For this review, take the finished solid that the model builds, in its own axes (mm). A direction names the side the tool comes from. Round coordinates to 2 decimals unless told otherwise and drop trailing zeros. Loops run counter-clockwise (first coordinate to the right, second up) from the corner with the lowest first, then second, coordinate; pieces in that order, holes last. Notation, with made-up numbers: M 41,51 L 78,51 A18 ccw 78,84 Z; hole C 13.5,-5.5 d2. An arc over 180 degrees is marked long. One line per question, with ' | ' between items. Start each with the question number.
1) We need section B-B (x = -10). Give the boundary of the cut face in (y, z).
2) We need section D-D (y = -2.5). Give the boundary of the cut face in (x, z), and give its area (3 significant figures).
3) We need section A-A (y = 3). Give the boundary of the cut face in (x, z), and give its area (3 significant figures).
4) We need section C-C (z = 5). Give the boundary of the cut face in (x, y), and give its area (3 significant figures).
5) Mouldability with a two-part tool opening along Y and no side actions: class faces 3 (the face through (5, 0, 8)), 4 (the face through (-14, 3, 5)), 5 (the face through (0, -11, 5)) as pulls with the +Y half, pulls with the -Y half, needs draft (parallel to the pull), parting line crosses it, or undercut.
6) For probe 1 along Y at (x, z) = (-10, 5); probe 2 along X at (y, z) = (2.25, 7.25); probe 3 along Z at (x, y) = (10.5, -8.75), list the stretches that pass through material, from the lowest coordinate up. Write a range as from..to.
7) For faces 1 (the face through (19, 0, 10)), 2 (the face through (13, 0, 8)), list the 3-axis set-ups (+Z, -Z, +X, -X, +Y, -Y) from which the entire face can be reached by the end or side of a thin tool; tool diameter is ignored.
```python
from build123d import *

# Parameters (mm, degrees)
SKETCH_1_W          = 50
SKETCH_1_H          = 22
EXTRUDE_1_DEPTH     = 10
SKETCH_2_R          = 4
CUT_EXTRUDE_1_DEPTH = 30.086079144
SKETCH_3_W          = 8
SKETCH_3_H          = 22
CUT_EXTRUDE_2_DEPTH = 4


with BuildPart() as part:
    # Эскиз1 → Бобышка-Вытянуть1 (new body)
    with BuildSketch(Plane.XY):
        Rectangle(SKETCH_1_W, SKETCH_1_H)
    extrude(amount=EXTRUDE_1_DEPTH)

    # Эскиз2 → Вырез-Вытянуть1 (cut, through all)
    with BuildSketch(Plane.XY.offset(10)):
        with Locations((-10, 3)):
            Circle(SKETCH_2_R)
    extrude(amount=-CUT_EXTRUDE_1_DEPTH, mode=Mode.SUBTRACT)

    # Эскиз3 → Вырез-Вытянуть2 (cut)
    with BuildSketch(Plane.XY.offset(10)):
        with Locations((9, 0)):
            Rectangle(SKETCH_3_W, SKETCH_3_H)
    extrude(amount=-CUT_EXTRUDE_2_DEPTH, mode=Mode.SUBTRACT)


solid = part.part
```
Answers below:
1) outline: M -11,0 L -1,0 L -1,10 L -11,10 Z; M 7,0 L 11,0 L 11,10 L 7,10 Z
2) outline: M -25,0 L 25,0 L 25,10 L 13,10 L 13,6 L 5,6 L 5,10 L -25,10 Z | area: 468 mm^2
3) outline: M -25,0 L -14,0 L -14,10 L -25,10 Z; M -6,0 L 25,0 L 25,10 L 13,10 L 13,6 L 5,6 L 5,10 L -6,10 Z | area: 388 mm^2
4) outline: M -25,-11 L 25,-11 L 25,11 L -25,11 Z; hole C -10,3 d8 | area: 1,050 mm^2
5) face 3: needs draft | face 4: undercut | face 5: pulls with the -Y half
6) probe 1: -11..-1, 7..11 | probe 2: -25..-13.93, -6.07..5, 13..25 | probe 3: 0..6
7) face 1: +Z, +X, -X, +Y, -Y | face 2: +Z, +Y, -Y
